Read the model definition and answer for the solid it produces. Units are mm, in the model's axes. Face numbers are marked on the shaded views. A direction names the side the tool comes from. Round coordinates to 2 decimals unless told otherwise and drop trailing zeros. Write each loop counter-clockwise with the first axis right and the second up, starting at its lowest first coordinate (ties: lowest second). Pieces come first, ordered by that corner, then holes. Notation, with made-up numbers: (24, 10.25) - (62, 10.25) arc R24 cw to (62, 48.25) - close; hole circle Ø9 at (-7, -29.75). An arc over 180 degrees is marked (long way). Answer as CSV lines item,"result". Start each with the question number.
1) Each of these flat-tipped pins is pushed along its axis until it touches: pin 1 (16 mm diameter, centred on x = 125, y = -7.5, fed in from +Z); pin 2 (8.5 mm diameter, centred on x = 127, z = -31.5, fed in from -Y); pin 3 (1 mm diameter, centred on y = -29, z = 6, fed in from -X). Where does it stop, or does it pass through?
2) For a pull along Z with two mould halves and no side action, classify the marked faces 1, 2 and 3 as +Z half, -Z half, draft (parallel to the pull), parting line (faces both ways), or undercut.
3) Which of the six approach directions +Z, -Z, +X, -X, +Y, -Y give full straight-line access (tool end or side, diameter ignored) to the marked faces 4 and 5?
4) Consider line 1 along Y through (x, z) = (117.5, 12.5); line 2 along X through (y, z) = (-32, 17); line 3 along Y through (x, z) = (130.5, -8.5). Determine where each line is inside the solid, lowest interval first.
5) Find section D-D on z = -15. Determine the outline of the cut face in (x, y).
6) Find section A-A on z = 12.5. Determine the outline of the cut face in (x, y), then the cut area to 3 significant figures.
from build123d import *

# Parameters (mm, degrees)
EXTRUDE_1_DEPTH      = 64
CUT_EXTRUDE_1_DEPTH  = 64
SKETCH_4_W           = 3
SKETCH_4_H           = 15
CUT_EXTRUDE_2_DEPTH  = 84
CUT_EXTRUDE_3_DEPTH  = 61
CUT_EXTRUDE_4_DEPTH  = 22
CUT_EXTRUDE_5_DEPTH  = 22
FILLET_1_R           = 3
SKETCH_8_R           = 1.5
CUT_EXTRUDE_8_DEPTH  = 10
CUT_EXTRUDE_9_DEPTH  = 13
SKETCH_10_R          = 1.5
CUT_EXTRUDE_10_DEPTH = 10
FILLET_2_R           = 3


with BuildPart() as part:
    # 草图2 → 凸台-拉伸1 (new body)
    with BuildSketch(Plane(origin=(0, 0, 0), x_dir=(1, 0, 0), z_dir=(0, 1, 0))):
        with BuildLine():
            Line((0, 0), (122.35155125, 57.053465335))
            ThreePointArc((122.35155125, 57.053465335), (134.052652215, 15.965163138), (132.328890593, -26.721989344))
            Line((132.328890593, -26.721989344), (0, 0))
        make_face()
    extrude(amount=-EXTRUDE_1_DEPTH)

    # 草图3 → 切除-拉伸1 (cut)
    with BuildSketch(Plane(origin=(0, 0, 0), x_dir=(1, 0, 0), z_dir=(0, 1, 0))):
        with BuildLine():
            Line((0, 0), (104.225395509, 48.6011001))
            ThreePointArc((104.225395509, 48.6011001), (114.193000035, 13.599953785), (112.724610505, -22.763176108))
            Line((112.724610505, -22.763176108), (0, 0))
        make_face()
    extrude(amount=-CUT_EXTRUDE_1_DEPTH, mode=Mode.SUBTRACT)

    # 草图4 → 切除-拉伸2 (cut)
    with BuildSketch(Plane(origin=(0, 0, 0), x_dir=(1, 0, 0), z_dir=(0, 1, 0))):
        with Locations((114.5, -12.5)):
            Rectangle(SKETCH_4_W, SKETCH_4_H)
    extrude(amount=-CUT_EXTRUDE_2_DEPTH, mode=Mode.SUBTRACT)

    # 草图5 → 切除-拉伸3 (cut)
    with BuildSketch(Plane.XZ.offset(64)):
        with BuildLine():
            Line((132.328890593, 26.721989344), (118.281412986, 23.885295518))
            ThreePointArc((118.281412986, 23.885295518), (118.656610088, 21.945589136), (119, 20))
            Line((119, 20), (119, 5))
            Line((119, 5), (117.894020205, 5))
            ThreePointArc((117.894020205, 5), (115.718279593, -23.092851014), (106.94431887, -49.868954885))
            Line((106.94431887, -49.868954885), (122.35155125, -57.053465335))
            ThreePointArc((122.35155125, -57.053465335), (134.052652215, -15.965163138), (132.328890593, 26.721989344))
        make_face()
    extrude(amount=-CUT_EXTRUDE_3_DEPTH, mode=Mode.SUBTRACT)

    # 草图6 → 切除-拉伸4 (cut)
    with BuildSketch(Plane(origin=(0, 0, 0), x_dir=(1, 0, 0), z_dir=(0, 1, 0))):
        with BuildLine():
            Line((135, 0), (115, 0))
            ThreePointArc((115, 0), (114.972810018, -2.500591226), (114.891252931, -5))
            Line((114.891252931, -5), (116, -5))
            Line((116, -5), (116, -20))
            Line((116, -20), (113.247516529, -20))
            ThreePointArc((113.247516529, -20), (112.994510197, -21.383186511), (112.724610505, -22.763176108))
            Line((112.724610505, -22.763176108), (132.328890593, -26.721989344))
            ThreePointArc((132.328890593, -26.721989344), (134.330562848, -13.427579268), (135, 0))
        make_face()
    extrude(amount=-CUT_EXTRUDE_4_DEPTH, mode=Mode.SUBTRACT)

    # 草图7 → 切除-拉伸5 (cut)
    with BuildSketch(Plane.XZ.offset(64)):
        with BuildLine():
            Line((116, 5), (119, 5))
            Line((119, 5), (119, 20))
            ThreePointArc((119, 20), (118.656610088, 21.945589136), (118.281412986, 23.885295518))
            Line((118.281412986, 23.885295518), (112.724610505, 22.763176108))
            ThreePointArc((112.724610505, 22.763176108), (112.994510197, 21.383186511), (113.247516529, 20))
            Line((113.247516529, 20), (116, 20))
            Line((116, 20), (116, 5))
        make_face()
    extrude(amount=-CUT_EXTRUDE_5_DEPTH, mode=Mode.SUBTRACT)

    # 圆角1
    fillet_1_edges = [part.edges().sort_by_distance(p)[0] for p in [
        (122.35155125, -1.5, -57.053465335),
    ]]
    fillet(fillet_1_edges, radius=FILLET_1_R)

    # 草图8 → 切除-拉伸8 (cut)
    with BuildSketch(Plane(origin=(119, 0, 0), x_dir=(0, 0, -1), z_dir=(1, 0, 0))):
        with Locations((-12.5, -27.5)):
            Circle(SKETCH_8_R)
        with Locations((-12.5, -36.5)):
            Circle(SKETCH_8_R)
    extrude(amount=-CUT_EXTRUDE_8_DEPTH, mode=Mode.SUBTRACT)

    # 草图9 → 切除-拉伸9 (cut)
    with BuildSketch(Plane.XZ.offset(64)):
        with BuildLine():
            Line((106.94431887, -49.868954885), (104.225395509, -48.6011001))
            ThreePointArc((104.225395509, -48.6011001), (112.788722348, -22.443353384), (114.891252931, 5))
            Line((114.891252931, 5), (117.894020205, 5))
            ThreePointArc((117.894020205, 5), (115.718279593, -23.092851014), (106.94431887, -49.868954885))
        make_face()
    extrude(amount=-CUT_EXTRUDE_9_DEPTH, mode=Mode.SUBTRACT)

    # 草图10 → 切除-拉伸10 (cut)
    with BuildSketch(Plane(origin=(0, 0, 0), x_dir=(1, 0, 0), z_dir=(0, 1, 0))):
        with Locations((121.091047045, 39.915013787)):
            Circle(SKETCH_10_R)
        with Locations((126.614572621, 15)):
            Circle(SKETCH_10_R)
    extrude(amount=-CUT_EXTRUDE_10_DEPTH, mode=Mode.SUBTRACT)

    # 圆角2
    fillet_2_edges = [part.edges().sort_by_distance(p)[0] for p in [
        (104.225395509, -25.5, -48.6011001),
    ]]
    fillet(fillet_2_edges, radius=FILLET_2_R)


solid = part.part
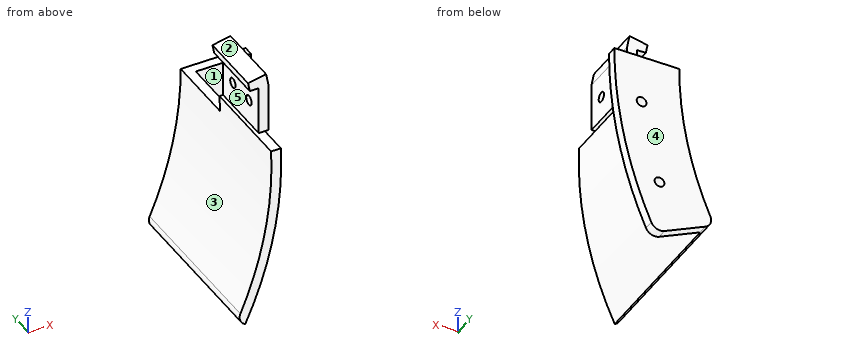
Check values:
1,pin 1,"stops at z = 0"
1,pin 2,"stops at y = -3"
1,pin 3,"stops at x = 116"
2,face 1,"draft"
2,face 2,"+Z half"
2,face 3,"undercut"
3,face 4,"+Z, -Z, +X, -X, +Y"
3,face 5,"-X, +Y, -Y"
4,line 1,"y = -42 to -38, -35 to -29, -26 to -22"
4,line 2,"x = 116 to 119"
4,line 3,"y = -3 to 0"
5,outline,"(114.02, -51) - (117.04, -51) - (117.04, -3) - (125.11, -3) - (125.11, 0) - (114.02, 0) - close; (128.11, -3) - (134.16, -3) - (134.16, 0) - (128.11, 0) - close"
6,outline,"(116, -42) - (119, -42) - (119, -38) - (116, -38) - close; (116, -35) - (119, -35) - (119, -29) - (116, -29) - close; (116, -26) - (119, -26) - (119, -22) - (116, -22) - close"
6,area,"42.0 mm^2"
